Geometry check sheet. Reference: the model listing, model coordinates, mm. Coordinates: 2 decimals unless noted, no trailing zeros. Order: outer loops, then holes, each group sorted by start corner. A loop starts at its lowest first (then second) coordinate and runs counter-clockwise, first axis right, second up. Notation, with made-up numbers: M -34,60 L -14,60 A25 ccw -14,89 Z; hole C 65.25,71.25 d7. An arc over 180 degrees is marked long. Use CSV: the item, a comma, the result in double quotes. Start each with the question number.
```python
from build123d import *

# Parameters (mm, degrees)
F0_R         = 21.5
F1_DEPTH     = 25
F2_T1_DEPTH  = 106
F2_T4_ANGLE  = 180
F2_T8_ANGLE  = 103.6596556564
F2_S9_R      = 30
F2_T10_DEPTH = 37
F2_T12_ANGLE = 180
F2_T14_ANGLE = 180
F2_T16_ANGLE = 180


# Not quite as in the source:
# - a fillet or chamfer that OpenCascade refuses, or shapes differently, is made with other operations: its cross-section is extruded or revolved along the edge and cut away or added


with BuildPart() as f1:
    # F0 (on Front) → F1 (new body)
    with BuildSketch(Plane.XZ):
        with BuildLine():
            ThreePointArc((14.0623611104, -26.5), (25.7086642332, -15.4617134673), (30, 0))
            ThreePointArc((30, 0), (25.7086642332, 15.4617134673), (14.0623611104, 26.5))
            ThreePointArc((14.0623611104, 26.5), (0, 23), (-14.0623611104, 26.5))
            ThreePointArc((-14.0623611104, 26.5), (-25.7086642332, 15.4617134673), (-30, 0))
            ThreePointArc((-30, 0), (-25.7086642332, -15.4617134673), (-14.0623611104, -26.5))
            ThreePointArc((-14.0623611104, -26.5), (0, -23), (14.0623611104, -26.5))
        make_face()
        Circle(F0_R, mode=Mode.SUBTRACT)
        with BuildLine():
            Line((30, -53), (30, 0))
            ThreePointArc((30, 0), (25.7086642332, -15.4617134673), (14.0623611104, -26.5))
            ThreePointArc((14.0623611104, -26.5), (25.7086642332, -37.5382865327), (30, -53))
        make_face()
        with BuildLine():
            ThreePointArc((14.0623611104, 26.5), (25.7086642332, 15.4617134673), (30, 0))
            Line((30, 0), (30, 53))
            ThreePointArc((30, 53), (25.7086642332, 37.5382865327), (14.0623611104, 26.5))
        make_face()
        with BuildLine():
            ThreePointArc((-14.0623611104, 26.5), (0, 30), (14.0623611104, 26.5))
            ThreePointArc((14.0623611104, 26.5), (25.7086642332, 37.5382865327), (30, 53))
            ThreePointArc((30, 53), (0, 83), (-30, 53))
            ThreePointArc((-30, 53), (-25.7086642332, 37.5382865327), (-14.0623611104, 26.5))
        make_face()
        with Locations((0, 53)):
            Circle(F0_R, mode=Mode.SUBTRACT)
        with BuildLine():
            ThreePointArc((30, -53), (25.7086642332, -37.5382865327), (14.0623611104, -26.5))
            ThreePointArc((14.0623611104, -26.5), (0, -30), (-14.0623611104, -26.5))
            ThreePointArc((-14.0623611104, -26.5), (-25.7086642332, -37.5382865327), (-30, -53))
            ThreePointArc((-30, -53), (0, -83), (30, -53))
        make_face()
        with Locations((0, -53)):
            Circle(F0_R, mode=Mode.SUBTRACT)
        with BuildLine():
            ThreePointArc((-30, 0), (-25.7086642332, 15.4617134673), (-14.0623611104, 26.5))
            ThreePointArc((-14.0623611104, 26.5), (-25.7086642332, 37.5382865327), (-30, 53))
            Line((-30, 53), (-30, 0))
        make_face()
        with BuildLine():
            ThreePointArc((-30, -53), (-25.7086642332, -37.5382865327), (-14.0623611104, -26.5))
            ThreePointArc((-14.0623611104, -26.5), (-25.7086642332, -15.4617134673), (-30, 0))
            Line((-30, 0), (-30, -53))
        make_face()
    extrude(amount=F1_DEPTH)

    # F2: fillet of radius 5 on 3 edges, made by hand

    # F2_s2 → F2_t1 (cut)
    with BuildSketch(Plane.XY.offset(-53)):
        with BuildLine():
            ThreePointArc((-30, -20), (-28.5355339059, -23.5355339059), (-25, -25))
            Line((-25, -25), (-25, -25.1))
            Line((-25, -25.1), (-30.1, -25.1))
            Line((-30.1, -25.1), (-30.1, -20))
            Line((-30.1, -20), (-30, -20))
        make_face()
        with BuildLine():
            ThreePointArc((-30, -5), (-28.5355339059, -1.4644660941), (-25, 0))
            Line((-25, 0), (-25, 0.1))
            Line((-25, 0.1), (-30.1, 0.1))
            Line((-30.1, 0.1), (-30.1, -5))
            Line((-30.1, -5), (-30, -5))
        make_face()
        with BuildLine():
            ThreePointArc((30, -5), (28.5355339059, -1.4644660941), (25, 0))
            Line((25, 0), (25, 0.1))
            Line((25, 0.1), (30.1, 0.1))
            Line((30.1, 0.1), (30.1, -5))
            Line((30.1, -5), (30, -5))
        make_face()
        with BuildLine():
            ThreePointArc((30, -20), (28.5355339059, -23.5355339059), (25, -25))
            Line((25, -25), (25, -25.1))
            Line((25, -25.1), (30.1, -25.1))
            Line((30.1, -25.1), (30.1, -20))
            Line((30.1, -20), (30, -20))
        make_face()
    extrude(amount=F2_T1_DEPTH, mode=Mode.SUBTRACT)

    # F2_s3 → F2_t4 (revolve, cut)
    with BuildSketch(Plane.XY.offset(-53)):
        with BuildLine():
            ThreePointArc((-30, -5), (-28.5355339059, -1.4644660941), (-25, 0))
            Line((-25, 0), (-25, 0.1))
            Line((-25, 0.1), (-30.1, 0.1))
            Line((-30.1, 0.1), (-30.1, -5))
            Line((-30.1, -5), (-30, -5))
        make_face()
    revolve(axis=Axis((0, 0, -53), (0, -1, 0)), revolution_arc=F2_T4_ANGLE, mode=Mode.SUBTRACT)


with BuildPart() as f2_tool6:
    # F2_s7 → F2_t8 (revolve)
    with BuildSketch(Plane(origin=(-25.7504646383, 0, -32.7580804495), x_dir=(0, 1, 0), z_dir=(-0.6179991993, 0, -0.7861787263))):
        with BuildLine():
            ThreePointArc((-5, 2.7539575651), (-1.4644660941, 1.289491471), (0, -2.2460424349))
            Line((0, -2.2460424349), (0.1, -2.2460424349))
            Line((0.1, -2.2460424349), (0.1, 2.8539575651))
            Line((0.1, 2.8539575651), (-5, 2.8539575651))
            Line((-5, 2.8539575651), (-5, 2.7539575651))
        make_face()
    revolve(axis=Axis((0, 0, -53), (0, 1, 0)), revolution_arc=F2_T8_ANGLE)

    # F2_s9 → F2_t10 (intersect, symmetric)
    with BuildSketch(Plane.XZ.offset(4.2)):
        Circle(F2_S9_R)
    extrude(amount=F2_T10_DEPTH, both=True, mode=Mode.INTERSECT)


with BuildPart() as f1_1:
    add(f1.part)

    # F2_t5: cut F2_tool6
    add(f2_tool6.part, mode=Mode.SUBTRACT)

    # F2_s11 → F2_t12 (revolve, cut)
    with BuildSketch(Plane.XY.offset(53)):
        with BuildLine():
            ThreePointArc((30, -5), (28.5355339059, -1.4644660941), (25, 0))
            Line((25, 0), (25, 0.1))
            Line((25, 0.1), (30.1, 0.1))
            Line((30.1, 0.1), (30.1, -5))
            Line((30.1, -5), (30, -5))
        make_face()
    revolve(axis=Axis((0, 0, 53), (0, -1, 0)), revolution_arc=F2_T12_ANGLE, mode=Mode.SUBTRACT)

    # F2_s13 → F2_t14 (revolve, cut)
    with BuildSketch(Plane.XY.offset(53)):
        with BuildLine():
            ThreePointArc((30, -20), (28.5355339059, -23.5355339059), (25, -25))
            Line((25, -25), (25, -25.1))
            Line((25, -25.1), (30.1, -25.1))
            Line((30.1, -25.1), (30.1, -20))
            Line((30.1, -20), (30, -20))
        make_face()
    revolve(axis=Axis((0, -25, 53), (0, -1, 0)), revolution_arc=F2_T14_ANGLE, mode=Mode.SUBTRACT)

    # F2_s15 → F2_t16 (revolve, cut)
    with BuildSketch(Plane.XY.offset(-53)):
        with BuildLine():
            ThreePointArc((-30, -20), (-28.5355339059, -23.5355339059), (-25, -25))
            Line((-25, -25), (-25, -25.1))
            Line((-25, -25.1), (-30.1, -25.1))
            Line((-30.1, -25.1), (-30.1, -20))
            Line((-30.1, -20), (-30, -20))
        make_face()
    revolve(axis=Axis((0, -25, -53), (0, -1, 0)), revolution_arc=F2_T16_ANGLE, mode=Mode.SUBTRACT)


solid = f1_1.part
```
1) Section check C-C on x = 4. State how many separate pieces and enclosed holes the cut face has, then the cut area to 3 significant figures.
2) Section check B-B on y = -9. Record the boundary of the cut face in (x, z).
3) Material ranges on line 1 along Z through (x, y) = (0, -11.75); line 2 along Z through (x, y) = (19.5, -9.25); line 3 along Z through (x, y) = (-4, -12.25), recorded low to high.
4) Gauge pin test, flat ends, axial feed: P1, Ø12, axis at x = 6, y = -17, coming from the +Z side; P2, Ø1.5, axis at x = 22.5, y = -14.5, coming from the -Z side; P3, Ø10, axis at x = 11.5, y = -21, coming from the -Z side; P4, Ø6, axis at y = -20.5, z = 11, coming from the -X side. Record the tip position at first contact, or that the pin passes through.
5) Section check A-A on z = 0. Record the boundary of the cut face in (x, y), then the cut area to 3 significant figures.
6) Draft check along Z on faces 1 (the face through (-0.66, -12.395, -82.993)), 2 (the face through (0, -15, -23)), 3 (the face through (-2.799, -12.325, 21.317)), 4 (the face through (29, -23, -1)). Enter one of: +Z half, -Z half, draft (parallel to the pull), parting line (faces both ways), or undercut.
Results are:
1,separate pieces,"6"
1,enclosed holes,"0"
1,area,"618 mm²"
2,outline,"M -30,-53 A30 ccw 30,-53 L 30,53 A30 ccw -30,53 Z; hole C 0,-53 d43; hole C 0,0 d43; hole C 0,53 d43; hole M -14.06,-26.5 A30 ccw 14.06,-26.5 A30 ccw Z; hole M -14.06,26.5 A30 ccw 14.06,26.5 A30 ccw Z"
3,line 1,"z = -83 to -74.5, -31.5 to -30, -23 to -21.5, 21.5 to 23, 30 to 31.5, 74.5 to 83"
3,line 2,"z = -75.8 to -62.06, -43.94 to -9.06, 9.06 to 43.94, 62.06 to 75.8"
3,line 3,"z = -82.73 to -74.12, -31.88 to -29.73, -23.27 to -21.12, 21.12 to 23.27, 29.73 to 31.88, 74.12 to 82.73"
4,P1,"stops at z = 83"
4,P2,"stops at z = -73.66"
4,P3,"stops at z = -82.27"
4,P4,"stops at x = -30"
5,outline,"M -30,-20 A5 ccw -25,-25 L -21.5,-25 L -21.5,0 L -25,0 A5 ccw -30,-5 Z; M 21.5,-25 L 25,-25 A5 ccw 30,-20 L 30,-5 A5 ccw 25,0 L 21.5,0 Z"
5,area,"404 mm²"
6,face 1,"-Z half"
6,face 2,"undercut"
6,face 3,"undercut"
6,face 4,"draft"
